from build123d import *

# Parameters (mm, degrees)
SKETCH1_R           = 10
SKETCH1_R_2         = 3.3
BOSS_EXTRUDE1_DEPTH = 10
BOSS_EXTRUDE2_START = 32
SKETCH3_R           = 18
SKETCH3_R_2         = 10
BOSS_EXTRUDE2_DEPTH = 32
CHAMFER1_SIZE       = 0.5


with BuildPart() as part:
    # Sketch1 → Boss-Extrude1 (new body)
    with BuildSketch(Plane(origin=(0, 0, 0), x_dir=(0, -1, 0), z_dir=(0, 0, 1))):
        with BuildLine():
            Line((-18.894443628, 22), (18.894443628, 22))
            ThreePointArc((18.894443628, 22), (29, 0), (18.894443628, -22))
            Line((18.894443628, -22), (-18.894443628, -22))
            ThreePointArc((-18.894443628, -22), (-29, 0), (-18.894443628, 22))
        make_face()
        with Locations(Location((0, 0, 0), (0, 0, 90))):
            Circle(SKETCH1_R, mode=Mode.SUBTRACT)
        with Locations(Location((-23.5, 0, 0), (0, 0, 90))):
            Circle(SKETCH1_R_2, mode=Mode.SUBTRACT)
        with Locations(Location((-16.617009358, 16.617009358, 0), (0, 0, 90))):
            Circle(SKETCH1_R_2, mode=Mode.SUBTRACT)
        with Locations(Location((16.617009358, 16.617009358, 0), (0, 0, 90))):
            Circle(SKETCH1_R_2, mode=Mode.SUBTRACT)
        with Locations(Location((23.5, 0, 0), (0, 0, 90))):
            Circle(SKETCH1_R_2, mode=Mode.SUBTRACT)
        with Locations(Location((16.617009358, -16.617009358, 0), (0, 0, 90))):
            Circle(SKETCH1_R_2, mode=Mode.SUBTRACT)
        with Locations(Location((-16.617009358, -16.617009358, 0), (0, 0, 90))):
            Circle(SKETCH1_R_2, mode=Mode.SUBTRACT)
    extrude(amount=BOSS_EXTRUDE1_DEPTH)

    # Sketch3 → Boss-Extrude2 (add)
    with BuildSketch(Plane(origin=(0, 0, 0), x_dir=(0, -1, 0), z_dir=(0, 0, -1)).offset(BOSS_EXTRUDE2_START)):
        with Locations(Location((0, 0, 0), (0, 0, 270))):
            Circle(SKETCH3_R)
        with Locations(Location((0, 0, 0), (0, 0, 270))):
            Circle(SKETCH3_R_2, mode=Mode.SUBTRACT)
    extrude(amount=-BOSS_EXTRUDE2_DEPTH)

    # Chamfer1
    chamfer1_edges = [part.edges().sort_by_distance(p)[0] for p in [
        (0, 29, 10),
        (-10, 0, 10),
        (-22, 0, 10),
        (-3.3, 23.5, 0),
        (-3.3, 23.5, 10),
        (13.317009358, 16.617009358, 0),
        (13.317009358, 16.617009358, 10),
        (13.317009358, -16.617009358, 0),
        (13.317009358, -16.617009358, 10),
        (-3.3, -23.5, 0),
        (-3.3, -23.5, 10),
        (-19.917009358, -16.617009358, 0),
        (-19.917009358, -16.617009358, 10),
        (-19.917009358, 16.617009358, 0),
        (-19.917009358, 16.617009358, 10),
        (0, -29, 10),
        (-18, 0, 0),
        (-18, 0, -32),
        (-10, 0, -32),
        (-22, 0, 0),
        (0, 29, 0),
        (22, 0, 0),
        (0, -29, 0),
        (22, 0, 10),
    ]]
    chamfer(chamfer1_edges, length=CHAMFER1_SIZE)


solid = part.part
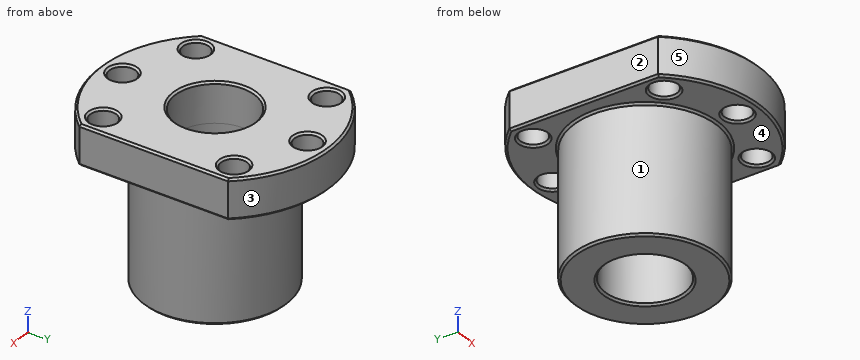
Input: part model. Units: mm. Frame: model coordinates. Face numbers are marked on the shaded views. A direction names the side the tool comes from. Coordinates: 2 decimals unless noted, no trailing zeros. Loops run counter-clockwise (first coordinate to the right, second up) from the corner with the lowest first, then second, coordinate; pieces in that order, holes last. Notation, with made-up numbers: (58, 5) -> (96, 5) arc R33 ccw to (96, 34) -> close; hole circle Ø1 at (43, 44.25). An arc over 180 degrees is marked (long way). Write item = value, one per line. Start each with the question number.
Item 1: Cut plane A-A, the plane y = 0. Return loops of the section in (x, z), plus the area to 3 significant figures.
Item 2: Cut plane D-D, the plane z = 4. Return loops of the section in (x, y), plus the area to 3 significant figures.
Item 3: Reachability of the marked faces 4 and 5 from +Z, -Z, +X, -X, +Y, -Y: full face, straight path, thin tool, end or side. Return the list, or none.
Item 4: Mould query, pull axis Y, two halves, no side actions, for the marked faces 1, 2 and 3. Classes: pulls with the +Y half, pulls with the -Y half, needs draft (parallel to the pull), parting line crosses it, or undercut.
Item 5: Material intervals for line 1 (Y direction, x = 0, z = -10.5); line 2 (Y direction, x = 14.5, z = 7); line 3 (Z direction, x = -20, y = 19), sorted ascending.
Item 6: First-contact query: P1, Ø4, axis at y = 12.5, z = -18.5, coming from the -X side; P2, Ø6, axis at x = 16.62, y = -16.62, coming from the -Z side; P3, Ø5, axis at x = -9.5, z = -18.5, coming from the -Y side; P4, Ø3, axis at x = -2, z = 2, coming from the -Y side. Flat tips, straight axial feed; report the tip coordinate or a pass-through.
Item 7: Cut plane B-B, the plane z = -3. Return loops of the section in (x, y).
Item 8: Cut plane C-C, the plane x = 0. Count the separate pieces of the cut face and the enclosed holes in it, plus the area to 3 significant figures.
Ans:
q1.outline = (-22, 0.5) -> (-21.5, 0) -> (-18.5, 0) -> (-18, -0.5) -> (-18, -31.5) -> (-17.5, -32) -> (-10.5, -32) -> (-10, -31.5) -> (-10, 9.5) -> (-10.5, 10) -> (-21.5, 10) -> (-22, 9.5) -> close; (10, -31.5) -> (10.5, -32) -> (17.5, -32) -> (18, -31.5) -> (18, -0.5) -> (18.5, 0) -> (21.5, 0) -> (22, 0.5) -> (22, 9.5) -> (21.5, 10) -> (10.5, 10) -> (10, 9.5) -> close
q1.area = 751 mm²
q2.outline = (-22, -18.89) arc R29 ccw to (22, -18.89) -> (22, 18.89) arc R29 ccw to (-22, 18.89) -> close; hole circle Ø6.6 at (-16.62, -16.62); hole circle Ø6.6 at (-16.62, 16.62); hole circle Ø20 at (0, 0); hole circle Ø6.6 at (0, -23.5); hole circle Ø6.6 at (0, 23.5); hole circle Ø6.6 at (16.62, -16.62); hole circle Ø6.6 at (16.62, 16.62)
q2.area = 1,760 mm²
q3.face_4 = -Z
q3.face_5 = +Z, -Z, -Y
q4.face_1 = parting line crosses it
q4.face_2 = needs draft
q4.face_3 = pulls with the +Y half
q5.line_1 = -18 to -10, 10 to 18
q5.line_2 = -25.11 to -19.15, -14.09 to 14.09, 19.15 to 25.11
q5.line_3 = 0 to 10
q6.P1 = -14.62
q6.P2 = through
q6.P3 = -16.58
q6.P4 = -29
q7.outline = circle Ø36 at (0, 0); hole circle Ø20 at (0, 0)
q8.separate_pieces = 4
q8.enclosed_holes = 0
q8.area = 758 mm²
